Geometry check sheet. Reference: drawing and pictorial views, mm from the part's lowest x, y, z. Give positions to 0.01 mm unless a question says otherwise; leave off trailing zeros. Write each loop counter-clockwise with the first axis right and the second up, starting at its lowest first coordinate (ties: lowest second). Pieces come first, ordered by that corner, then holes. Notation, with made-up numbers: (75, 9.25) -> (127, 9.25) arc R18 cw to (127, 17.25) -> close; hole circle Ø10 at (71, 55). An arc over 180 degrees is marked (long way). Return JSON: item names as keys, results as strings.
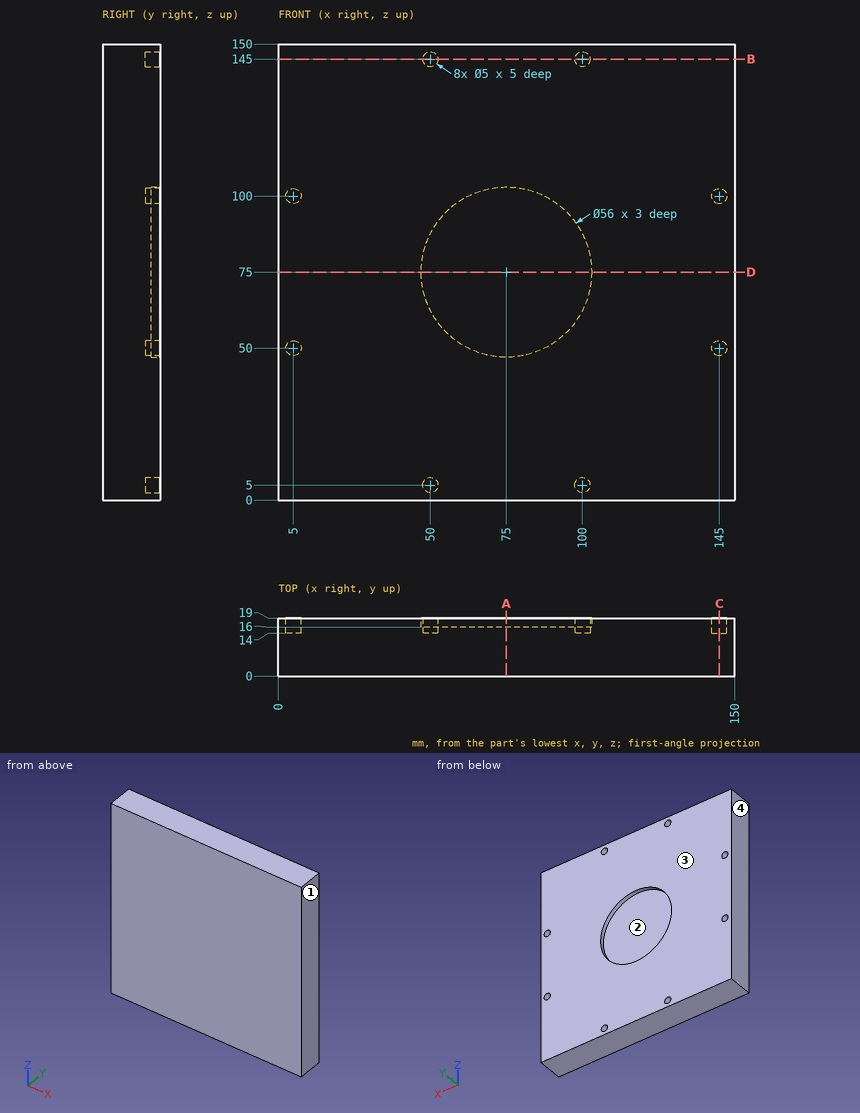
(1) Depth check by flat-ended pin: pin 1 Ø1.5 at (x, z) = (4, 100.5) entering from +Y. Enter the tip coordinate at first touch or a pass-through.
Reply:
{"pin 1": "y = 14"}
(2) Cross-section at D-D on z = 75. Enter the section's corners in (x, y).
Reply:
{"outline": "(0, 0) -> (150, 0) -> (150, 19) -> (103, 19) -> (103, 16) -> (47, 16) -> (47, 19) -> (0, 19) -> close"}
(3) Cross-section at C-C on x = 145. Enter the section's corners in (y, z), then the cut area to 3 significant figures.
Reply:
{"outline": "(0, 0) -> (19, 0) -> (19, 47.5) -> (14, 47.5) -> (14, 52.5) -> (19, 52.5) -> (19, 97.5) -> (14, 97.5) -> (14, 102.5) -> (19, 102.5) -> (19, 150) -> (0, 150) -> close", "area": "2,800 mm^2"}
(4) Cross-section at B-B on z = 145. Enter the section's corners in (x, y), then the cut area to 3 significant figures.
Reply:
{"outline": "(0, 0) -> (150, 0) -> (150, 19) -> (102.5, 19) -> (102.5, 14) -> (97.5, 14) -> (97.5, 19) -> (52.5, 19) -> (52.5, 14) -> (47.5, 14) -> (47.5, 19) -> (0, 19) -> close", "area": "2,800 mm^2"}
(5) Thickness scan on L1, parallel to X at y = 15.9, z = 50; L2, parallel to X at y = 15.05, z = 145; L3, parallel to Z at x = 75, y = 17.8. Record the ranges inside material, lowest first.
Reply:
{"L1": "0 to 2.5, 7.5 to 142.5, 147.5 to 150", "L2": "0 to 47.5, 52.5 to 97.5, 102.5 to 150", "L3": "0 to 47, 103 to 150"}
(6) Cross-section at A-A on x = 75. Enter the section's corners in (y, z).
Reply:
{"outline": "(0, 0) -> (19, 0) -> (19, 47) -> (16, 47) -> (16, 103) -> (19, 103) -> (19, 150) -> (0, 150) -> close"}
(7) Release check for a two-part mould opening along X. For the marked faces 1, 2, 3 and 4 record: pulls with the +X half, pulls with the -X half, needs draft (parallel to the pull), parting line crosses it, or undercut.
Reply:
{"face 1": "pulls with the +X half", "face 2": "undercut", "face 3": "needs draft", "face 4": "pulls with the -X half"}
